The listing builds one solid part. Answer for the finished solid, in the listing's coordinates (mm). Face numbers are marked on the shaded views. A direction names the side the tool comes from. Give positions to 0.01 mm unless a question says otherwise; leave off trailing zeros. Order: outer loops, then holes, each group sorted by start corner. A loop starts at its lowest first (then second) coordinate and runs counter-clockwise, first axis right, second up. Notation, with made-up numbers: (-14.5, 33) -> (18.5, 33) arc R11 ccw to (18.5, 41) -> close; hole circle Ø10 at (-16, 32). An arc over 180 degrees is marked (long way). Answer as a JSON object with one key per item and string values. Group by question number.
```python
from build123d import *

# Parameters (mm, degrees)
F0_R      = 7
F1_DEPTH  = 28.8
F4_DEPTH  = 12
F6_DEPTH  = 10
F8_DEPTH  = 10
F9_R      = 3.4
F10_DEPTH = 12
F11_R     = 2
F12_R     = 4


with BuildPart() as f1:
    # F0 (on Front) → F1 (new body)
    with BuildSketch(Plane.XZ):
        with BuildLine():
            Line((100, 0), (12, 0))
            ThreePointArc((12, 0), (-8.4852813742, 8.4852813742), (0, -12))
            Line((0, -12), (100, -12))
            Line((100, -12), (100, 0))
        make_face()
        Circle(F0_R, mode=Mode.SUBTRACT)
    extrude(amount=F1_DEPTH)

    # F3 (on offset) → F4 (cut)
    with BuildSketch(Plane.XZ.offset(20.4)):
        with BuildLine():
            Line((14, -12), (14, 0))
            Line((14, 0), (12, 0))
            ThreePointArc((12, 0), (-8.4852813742, 8.4852813742), (0, -12))
            Line((0, -12), (14, -12))
        make_face()
    extrude(amount=-F4_DEPTH, mode=Mode.SUBTRACT)

    # F5 (on face) → F6 (join)
    with BuildSketch(Plane.XZ.offset(28.8)):
        with BuildLine():
            Line((57.36, 0), (65, 0))
            Line((65, 0), (75, 0))
            Line((75, 0), (75, 20))
            Line((75, 20), (65, 20))
            ThreePointArc((65, 20), (63.0248532563, 9.2952660561), (57.36, 0))
        make_face()
    extrude(amount=-F6_DEPTH)

    # F7 (on face) → F8 (cut, through all)
    with BuildSketch(Plane.XZ.offset(28.8)):
        Polygon((57.36, -12), (57.36, 0), (42.36, 0), (47.36, -12), align=None)
    extrude(amount=-F8_DEPTH, mode=Mode.SUBTRACT)

    # F9 (on face) → F10 (cut, through all)
    with BuildSketch(Plane.XY):
        with Locations((77, -9.4)):
            Circle(F9_R)
    extrude(amount=-F10_DEPTH, mode=Mode.SUBTRACT)

    # F11
    f11_edges = [f1.edges().sort_by_distance(p)[0] for p in [
        (75, -23.8, 0),
        (12, -24.6, 0),
        (12, -4.2, 0),
    ]]
    fillet(f11_edges, radius=F11_R)

    # F12
    f12_edges = [f1.edges().sort_by_distance(p)[0] for p in [
        (75, -23.8, 20),
        (100, -14.4, 0),
    ]]
    fillet(f12_edges, radius=F12_R)


solid = f1.part
```
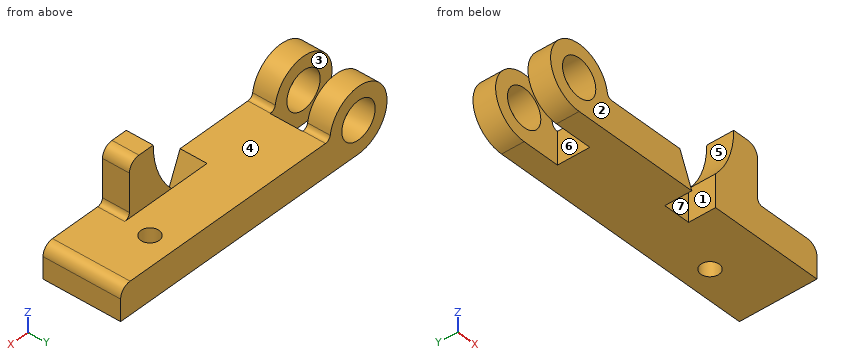
(1) A cutting plane is placed at D-D (z = 10). Determine the outline of the cut face in (x, y), and give its area (3 significant figures).
(2) Flat-ended cylindrical pins translate along their axes: pin 1 Ø3 at (y, z) = (-23.5, -6.5) entering from -X; pin 2 Ø8 at (y, z) = (-23.5, 10) entering from +X; pin 3 Ø1 at (x, y) = (66.5, -15) entering from +Z; pin 4 Ø12.5 at (x, z) = (0, 0) entering from +Y. Find the tip coordinate at first contact, or state that the pin passes through.
(3) Find the intervals of material crossed by line 1 along Z through (x, y) = (0, -23.25); line 2 along X through (y, z) = (-24.5, -5); line 3 along Y through (x, z) = (77, -8), in increasing order. Write a range as [from, to].
(4) Which of the six approach directions +Z, -Z, +X, -X, +Y, -Y give full straight-line access (tool end or side, diameter ignored) to the marked faces 4, 5, 6 and 7?
(5) A cutting plane is placed at B-B (y = -3.5). Determine the outline of the cut face in (x, z).
(6) For a pull along Y with two mould halves and no side action, classify the marked faces 1, 2 and 3 as +Y half, -Y half, draft (parallel to the pull), parting line (faces both ways), or undercut.
(7) A cutting plane is placed at C-C (z = -3). Determine the outline of the cut face in (x, y), and give its area (3 significant figures).
(8) A cutting plane is placed at A-A (y = -23). Determine the outline of the cut face in (x, z).
Check sheet entries:
{
 "1": {"outline": "(-6.63, -28.8) -> (6.63, -28.8) -> (6.63, -20.4) -> (-6.63, -20.4) -> close; (-6.63, -8.4) -> (6.63, -8.4) -> (6.63, 0) -> (-6.63, 0) -> close; (63.28, -28.8) -> (75, -28.8) -> (75, -18.8) -> (63.28, -18.8) -> close", "area": "340 mm2"},
 "2": {"pin 1": "stops at x = -10.91", "pin 2": "stops at x = 75", "pin 3": "stops at z = 0", "pin 4": "passes through"},
 "3": {"line 1": "z = [-12, -7], [7, 12]", "line 2": "x = [-10.91, -4.9], [4.9, 44.44], [57.36, 100]", "line 3": "y = [-28.8, -12.8], [-6, 0]"},
 "4": {"face 4": "+Z, +Y", "face 5": "+Z, +Y, -Y", "face 6": "+Z, -Z, -X", "face 7": "+Z, -Y"},
 "5": {"outline": "(0, -12) -> (100, -12) -> (100, -4) arc R4 ccw to (96, 0) -> (13.86, 0) arc R2 cw to (11.88, 1.71) arc R12 ccw (long way) to start; hole circle Ø14 at (0, 0)"},
 "6": {"face 1": "draft", "face 2": "-Y half", "face 3": "undercut"},
 "7": {"outline": "(-11.62, -28.8) -> (-6.32, -28.8) -> (-6.32, -20.4) -> (-11.62, -20.4) -> close; (-11.62, -8.4) -> (-6.32, -8.4) -> (-6.32, 0) -> (-11.62, 0) -> close; (6.32, -28.8) -> (43.61, -28.8) -> (43.61, -18.8) -> (57.36, -18.8) -> (57.36, -28.8) -> (99.87, -28.8) -> (99.87, 0) -> (6.32, 0) -> (6.32, -8.4) -> (14, -8.4) -> (14, -20.4) -> (6.32, -20.4) -> close; hole circle Ø6.8 at (77, -9.4)", "area": "2,520 mm2"},
 "8": {"outline": "(0, -12) -> (47.36, -12) -> (42.36, 0) -> (13.86, 0) arc R2 cw to (11.88, 1.71) arc R12 ccw (long way) to start; (57.36, -12) -> (100, -12) -> (100, -4) arc R4 ccw to (96, 0) -> (77, 0) arc R2 cw to (75, 2) -> (75, 16) arc R4 ccw to (71, 20) -> (65, 20) arc R30 cw to (57.36, 0) -> close; hole circle Ø14 at (0, 0)"}
}
